Geometry: final body of the model. Coordinates: model frame, mm. Face numbers are marked on the shaded views. A direction names the side the tool comes from. Round coordinates to 2 decimals unless told otherwise and drop trailing zeros. Write each loop counter-clockwise with the first axis right and the second up, starting at its lowest first coordinate (ties: lowest second). Pieces come first, ordered by that corner, then holes. Notation, with made-up numbers: M 69.5,22 L 78.5,22 A24 cw 78.5,38 Z; hole C -2,29.25 d1. An arc over 180 degrees is marked long. Put each result on its own line as item: value. Start each with the question number.
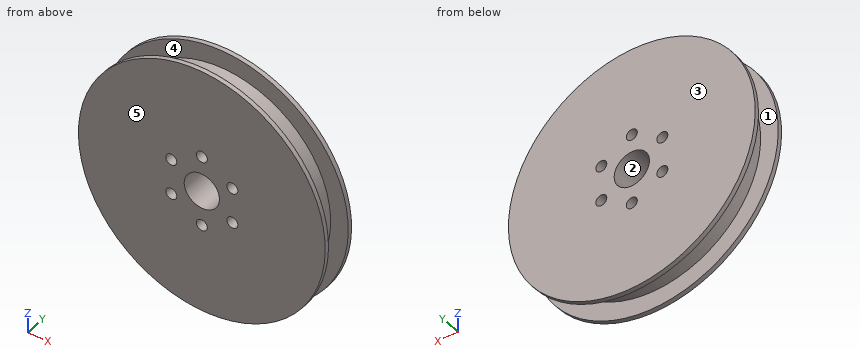
```python
from build123d import *

# Parameters (mm, degrees)
SKETCH2_R           = 76.2
SKETCH2_R_2         = 3.96875
SKETCH2_R_3         = 12.7
BOSS_EXTRUDE1_DEPTH = 19.05
SKETCH3_R           = 88.9
SKETCH3_R_2         = 3.96875
SKETCH3_R_3         = 12.7
BOSS_EXTRUDE2_DEPTH = 3.175
BOSS_EXTRUDE3_START = 3.175
SKETCH4_R           = 88.9
SKETCH4_R_2         = 12.7
SKETCH4_R_3         = 3.96875
BOSS_EXTRUDE3_DEPTH = 3.175


with BuildPart() as part:
    # Sketch2 → Boss-Extrude1 (new body)
    with BuildSketch(Plane(origin=(0, 0, 0), x_dir=(1, 0, 0), z_dir=(0, 1, 0))):
        with Locations(Location((0, 0, 0), (0, 0, 90))):
            Circle(SKETCH2_R)
        with Locations(Location((0, 25.4, 0), (0, 0, 90))):
            Circle(SKETCH2_R_2, mode=Mode.SUBTRACT)
        with Locations(Location((21.997045256, 12.7, 0), (0, 0, 90))):
            Circle(SKETCH2_R_2, mode=Mode.SUBTRACT)
        with Locations(Location((21.997045256, -12.7, 0), (0, 0, 90))):
            Circle(SKETCH2_R_2, mode=Mode.SUBTRACT)
        with Locations(Location((0, -25.4, 0), (0, 0, 90))):
            Circle(SKETCH2_R_2, mode=Mode.SUBTRACT)
        with Locations(Location((-21.997045256, -12.7, 0), (0, 0, 90))):
            Circle(SKETCH2_R_2, mode=Mode.SUBTRACT)
        with Locations(Location((-21.997045256, 12.7, 0), (0, 0, 90))):
            Circle(SKETCH2_R_2, mode=Mode.SUBTRACT)
        with Locations(Location((0, 0, 0), (0, 0, 90))):
            Circle(SKETCH2_R_3, mode=Mode.SUBTRACT)
    extrude(amount=BOSS_EXTRUDE1_DEPTH)

    # Sketch3 → Boss-Extrude2 (add)
    with BuildSketch(Plane(origin=(0, 19.05, 0), x_dir=(1, 0, 0), z_dir=(0, 1, 0))):
        with Locations(Location((0, 0, 0), (0, 0, 270))):
            Circle(SKETCH3_R)
        with Locations(Location((0, 25.4, 0), (0, 0, 90))):
            Circle(SKETCH3_R_2, mode=Mode.SUBTRACT)
        with Locations(Location((21.997045256, 12.7, 0), (0, 0, 90))):
            Circle(SKETCH3_R_2, mode=Mode.SUBTRACT)
        with Locations(Location((21.997045256, -12.7, 0), (0, 0, 90))):
            Circle(SKETCH3_R_2, mode=Mode.SUBTRACT)
        with Locations(Location((0, -25.4, 0), (0, 0, 90))):
            Circle(SKETCH3_R_2, mode=Mode.SUBTRACT)
        with Locations(Location((-21.997045256, -12.7, 0), (0, 0, 90))):
            Circle(SKETCH3_R_2, mode=Mode.SUBTRACT)
        with Locations(Location((0, 0, 0), (0, 0, 90))):
            Circle(SKETCH3_R_3, mode=Mode.SUBTRACT)
        with Locations(Location((-21.997045256, 12.7, 0), (0, 0, 90))):
            Circle(SKETCH3_R_2, mode=Mode.SUBTRACT)
    extrude(amount=BOSS_EXTRUDE2_DEPTH)

    # Sketch4 → Boss-Extrude3 (add)
    with BuildSketch(Plane.XZ.offset(BOSS_EXTRUDE3_START)):
        with Locations(Location((0, 0, 0), (0, 0, 90))):
            Circle(SKETCH4_R)
        with Locations(Location((0, 0, 0), (0, 0, 270))):
            Circle(SKETCH4_R_2, mode=Mode.SUBTRACT)
        with Locations(Location((-21.997045256, -12.7, 0), (0, 0, 270))):
            Circle(SKETCH4_R_3, mode=Mode.SUBTRACT)
        with Locations(Location((0, -25.4, 0), (0, 0, 270))):
            Circle(SKETCH4_R_3, mode=Mode.SUBTRACT)
        with Locations(Location((21.997045256, -12.7, 0), (0, 0, 270))):
            Circle(SKETCH4_R_3, mode=Mode.SUBTRACT)
        with Locations(Location((21.997045256, 12.7, 0), (0, 0, 270))):
            Circle(SKETCH4_R_3, mode=Mode.SUBTRACT)
        with Locations(Location((0, 25.4, 0), (0, 0, 270))):
            Circle(SKETCH4_R_3, mode=Mode.SUBTRACT)
        with Locations(Location((-21.997045256, 12.7, 0), (0, 0, 270))):
            Circle(SKETCH4_R_3, mode=Mode.SUBTRACT)
    extrude(amount=-BOSS_EXTRUDE3_DEPTH)


solid = part.part
```
1) Access query for the marked faces 1 and 2. Directions: +Z, -Z, +X, -X, +Y, -Y. A direction counts if a zero-diameter tool reaches every point of the face in a straight line with its end or side. Return the directions, or none.
2) Section A-A, the plane x = 0. Output: boundary loops of the cut face in (y, z) (3 decimals).
3) Ray query, probe 1 along X at (y, z) = (2.5, 0); probe 2 along Z at (x, y) = (-23.5, 12); probe 3 along Y at (x, z) = (71, -42) (3 decimals). Return the intervals inside material, ascending.
4) First-contact query: pin 1 (7 mm diameter, centred on x = 22, z = 12.7, fed in from -Y); pin 2 (10 mm diameter, centred on x = -39, y = 4.5, fed in from -Z); pin 3 (4 mm diameter, centred on x = 69, y = 7, fed in from -Z); pin 4 (12 mm diameter, centred on y = 8, z = -62, fed in from -X). Flat tips, straight axial feed; report the tip coordinate or a pass-through.
5) Section B-B, the plane z = -25.4. Output: boundary loops of the cut face in (x, y) (3 decimals).
6) Section D-D, the plane z = 53. Output: boundary loops of the cut face in (x, y) (3 decimals), and give its area (3 significant figures).
7) Section C-C, the plane y = 2.5. Output: boundary loops of the cut face in (x, z), and give its area (3 significant figures).
8) Draft query along Y for the marked faces 3, 4 and 5. Return one class per face: +Y half, -Y half, draft (parallel to the pull), parting line (faces both ways), or undercut.
Solved:
1. face 1: none
1. face 2: +Y, -Y
2. outline: M -3.175,-88.9 L 0,-88.9 L 0,-76.2 L 19.05,-76.2 L 19.05,-88.9 L 22.225,-88.9 L 22.225,-29.369 L -3.175,-29.369 Z; M -3.175,-21.431 L 22.225,-21.431 L 22.225,-12.7 L -3.175,-12.7 Z; M -3.175,12.7 L 22.225,12.7 L 22.225,21.431 L -3.175,21.431 Z; M -3.175,29.369 L 22.225,29.369 L 22.225,88.9 L 19.05,88.9 L 19.05,76.2 L 0,76.2 L 0,88.9 L -3.175,88.9 Z
3. probe 1: x = -76.2 to -12.7, 12.7 to 76.2
3. probe 2: z = -72.49 to -16.37, -9.03 to 9.03, 16.37 to 72.49
3. probe 3: y = -3.175 to 0, 19.05 to 22.225
4. pin 1: passes through
4. pin 2: stops at z = -80.92
4. pin 3: stops at z = -36.3
4. pin 4: stops at x = -51.68
5. outline: M -85.194,-3.175 L -3.969,-3.175 L -3.969,22.225 L -85.194,22.225 L -85.194,19.05 L -71.842,19.05 L -71.842,0 L -85.194,0 Z; M 3.969,-3.175 L 85.194,-3.175 L 85.194,0 L 71.842,0 L 71.842,19.05 L 85.194,19.05 L 85.194,22.225 L 3.969,22.225 Z
6. outline: M -71.374,-3.175 L 71.374,-3.175 L 71.374,0 L 54.749,0 L 54.749,19.05 L 71.374,19.05 L 71.374,22.225 L -71.374,22.225 L -71.374,19.05 L -54.749,19.05 L -54.749,0 L -71.374,0 Z
6. area: 2,990 mm2
7. outline: C 0,0 d152.4; hole C -22,-12.7 d7.94; hole C -22,12.7 d7.94; hole C 0,0 d25.4; hole C 0,-25.4 d7.94; hole C 0,25.4 d7.94; hole C 22,-12.7 d7.94; hole C 22,12.7 d7.94
7. area: 17,400 mm2
8. face 3: +Y half
8. face 4: undercut
8. face 5: -Y half
